from build123d import *

# Parameters (mm, degrees)
F1_DEPTH = 80
F3_D     = 4
F5_D     = 4


with BuildPart() as f1:
    # F0 (on Front) → F1 (new body)
    with BuildSketch(Plane.XZ):
        Polygon((-83.770444, 112.477971), (-85.270444, 112.477971), (-85.270444, 32.477971), (-40.270444, 32.477971), (-40.270444, 33.977971), (-83.770444, 33.977971), align=None)
    extrude(amount=F1_DEPTH)

    # F3 (through all)
    with Locations(Plane(origin=(0, 0, 32.477971), x_dir=(1, 0, 0), z_dir=(0, 0, -1))):
        with Locations((-45.270444, 74), (-69.270444, 74), (-69.270444, 56), (-45.270444, 56), (-45.270444, 24), (-45.270444, 6), (-69.270444, 6), (-69.270444, 24)):
            Hole(F3_D / 2)

    # F5 (through all)
    with Locations(Plane(origin=(-85.270444, 0, 0), x_dir=(0, -1, 0), z_dir=(-1, 0, 0))):
        with Locations((20, 52.477971), (60, 52.477971), (60, 92.477971), (20, 92.477971)):
            Hole(F5_D / 2)


solid = f1.part
The listing builds one solid part. Answer for the finished solid, in the listing's coordinates (mm). A direction names the side the tool comes from. Give positions to 0.01 mm unless a question says otherwise; leave off trailing zeros. Loops run counter-clockwise (first coordinate to the right, second up) from the corner with the lowest first, then second, coordinate; pieces in that order, holes last. Notation, with made-up numbers: M -40,21.25 L -34,21.25 A23 cw -34,31.25 Z; hole C 65,-13 d2. An arc over 180 degrees is marked long. Answer as CSV lines item,"result".
Item 1: Straight lines are drawn through the part: line 1 along X through (y, z) = (-56, 33.55); line 2 along Z through (x, y) = (-84.8, -20); line 3 along X through (y, z) = (-16, 37). For each, find the intervals that lie inside material, in ascending order. Write a range as [from, to].
Values follow:
line 1,"x = [-85.27, -71.27], [-67.27, -47.27], [-43.27, -40.27]"
line 2,"z = [32.48, 50.48], [54.48, 90.48], [94.48, 112.48]"
line 3,"x = [-85.27, -83.77]"
Item 2: The part is cut by section D-D (z = 80). Give the vertices of the cut face in (x, y).
Values follow:
outline,"M -85.27,-80 L -83.77,-80 L -83.77,0 L -85.27,0 Z"
Item 3: The part is cut by section C-C (x = -63). Give the vertices of the cut face in (y, z), and give its area (3 significant figures).
Values follow:
outline,"M -80,32.48 L 0,32.48 L 0,33.98 L -80,33.98 Z"
area,"120 mm^2"
Item 4: The part is cut by section A-A (y = -24). Give the vertices of the cut face in (x, z), and give its area (3 significant figures).
Values follow:
outline,"M -85.27,32.48 L -71.27,32.48 L -71.27,33.98 L -83.77,33.98 L -83.77,112.48 L -85.27,112.48 Z; M -67.27,32.48 L -47.27,32.48 L -47.27,33.98 L -67.27,33.98 Z; M -43.27,32.48 L -40.27,32.48 L -40.27,33.98 L -43.27,33.98 Z"
area,"173 mm^2"
Item 5: The part is cut by section B-B (y = -67). Give the vertices of the cut face in (x, z), and give its area (3 significant figures).
Values follow:
outline,"M -85.27,32.48 L -40.27,32.48 L -40.27,33.98 L -83.77,33.98 L -83.77,112.48 L -85.27,112.48 Z"
area,"185 mm^2"
Item 6: Given pin 1 Ø3 at (y, z) = (-20, 52.48) entering from +X; pin 2 Ø5 at (x, y) = (-69.27, -74) entering from +Z; pin 3 Ø1.5 at (y, z) = (-27, 56.5) entering from +X, each flat-ended and moving along its own axis, determine where each tip first touches the part or whether it passes through.
Values follow:
pin 1,"passes through"
pin 2,"stops at z = 33.98"
pin 3,"stops at x = -83.77"
Item 7: The mould has two halves that part along X. Classify faces 3 (the flat face through (-83.77, -39, 73)), 4 (the flat face through (-85.27, -39, 73)), 5 (the cylindrical face through (-47.18, -6.6, 33.24)), 6 (the flat face through (-85, -80, 73)): released by +X, released by -X, zero draft, split by the parting line, or undercut.
Values follow:
face 3,"released by +X"
face 4,"released by -X"
face 5,"undercut"
face 6,"zero draft"
Item 8: Which of the six approach directions +Z, -Z, +X, -X, +Y, -Y give full straight-line access (tool end or side, diameter ignored) to faces 1 (the flat face through (-62, -39, 33.978)), 2 (the cylindrical face through (-67.272, -6.088, 33.238))?
Values follow:
face 1,"+Z, +X, +Y, -Y"
face 2,"+Z, -Z"
